Model file for the job. Use its own axes, mm. A direction names the side the tool comes from. Give positions to 0.01 mm unless a question says otherwise; leave off trailing zeros. Write each loop counter-clockwise with the first axis right and the second up, starting at its lowest first coordinate (ties: lowest second). Pieces come first, ordered by that corner, then holes. Notation, with made-up numbers: (32, 27) - (52, 27) arc R11 cw to (52, 37) - close; hole circle Ø8 at (70, -16.75). An arc over 180 degrees is marked (long way). Use a Markdown table: item, result. Add a question column.
```python
from build123d import *

# Parameters (mm, degrees)
F0_R     = 31.75
F1_DEPTH = 4.7625
F2_R     = 25.4
F3_DEPTH = 50.8
F5_D     = 41.275


with BuildPart() as f1:
    # F0 (on Right) → F1 (new body)
    with BuildSketch(Plane.YZ):
        Circle(F0_R)
    extrude(amount=F1_DEPTH)

    # F2 (on face) → F3 (join)
    with BuildSketch(Plane(origin=(0, 0, 0), x_dir=(0, -1, 0), z_dir=(-1, 0, 0))):
        Circle(F2_R)
    extrude(amount=-F3_DEPTH)

    # F5 (through all)
    with Locations(Plane.YZ.offset(50.8)):
        with Locations((0, 0)):
            Hole(F5_D / 2)


solid = f1.part
```
(1) Band-saw the part on C-C (x = 12). Write the cut outline in (y, z) (1 decimal), then the cut area to 3 significant figures.
(2) Which spindle directions (+Z, -Z, +X, -X, +Y, -Y) get a long thin tool onto all of the face, cutting with end or side? Do faces 4 (the flat face through (4.762, -14.3, 21.3)), 5 (the cylindrical face through (2.348, -6.883, -30.995)). Say none if no direction does.
(3) Band-saw the part on A-A (y = 0). Write the cut outline in (x, z).
(4) Probe probe 1 along Z at (x, y) = (34.5, 0); probe 2 along Z at (x, y) = (31, -16.5); probe 3 along X at (y, z) = (3.5, 29.5). List the from-to ranges inside material, lowest first. Write a range as [from, to].
(5) Two-plate mould, pull along Y, no slides. Class faces 1 (the flat face through (0, -21, 0)), 2 (the cylindrical face through (25.044, 4.474, -20.147)), 3 (the cylindrical face through (27.459, 5.506, -24.796)): +Y half, -Y half, draft (parallel to the pull), parting line (faces both ways), or undercut.
(6) Flat gauge pins, fed straight in: pin 1 (5 mm diameter, centred on x = 28, z = 8.5, fed in from +Y); pin 2 (4 mm diameter, centred on x = 12.5, y = -21, fed in from -Z); pin 3 (1.5 mm diameter, centred on x = 8.5, z = -5, fed in from +Y). Where does each tip first touch, or does it go through?
Model answer:
| question | item | result |
|---|---|---|
| 1 | outline | circle Ø50.8 at (0, 0); hole circle Ø41.3 at (0, 0) |
| 1 | area | 689 mm^2 |
| 2 | face 4 | +X |
| 2 | face 5 | +X, -X |
| 3 | outline | (0, -31.75) - (4.76, -31.75) - (4.76, -25.4) - (50.8, -25.4) - (50.8, -20.64) - (0, -20.64) - close; (0, 20.64) - (50.8, 20.64) - (50.8, 25.4) - (4.76, 25.4) - (4.76, 31.75) - (0, 31.75) - close |
| 4 | probe 1 | z = [-25.4, -20.64], [20.64, 25.4] |
| 4 | probe 2 | z = [-19.31, -12.4], [12.4, 19.31] |
| 4 | probe 3 | x = [0, 4.76] |
| 5 | face 1 | draft |
| 5 | face 2 | undercut |
| 5 | face 3 | parting line |
| 6 | pin 1 | stops at y = 24.68 |
| 6 | pin 2 | stops at z = -16.86 |
| 6 | pin 3 | stops at y = 25.04 |
